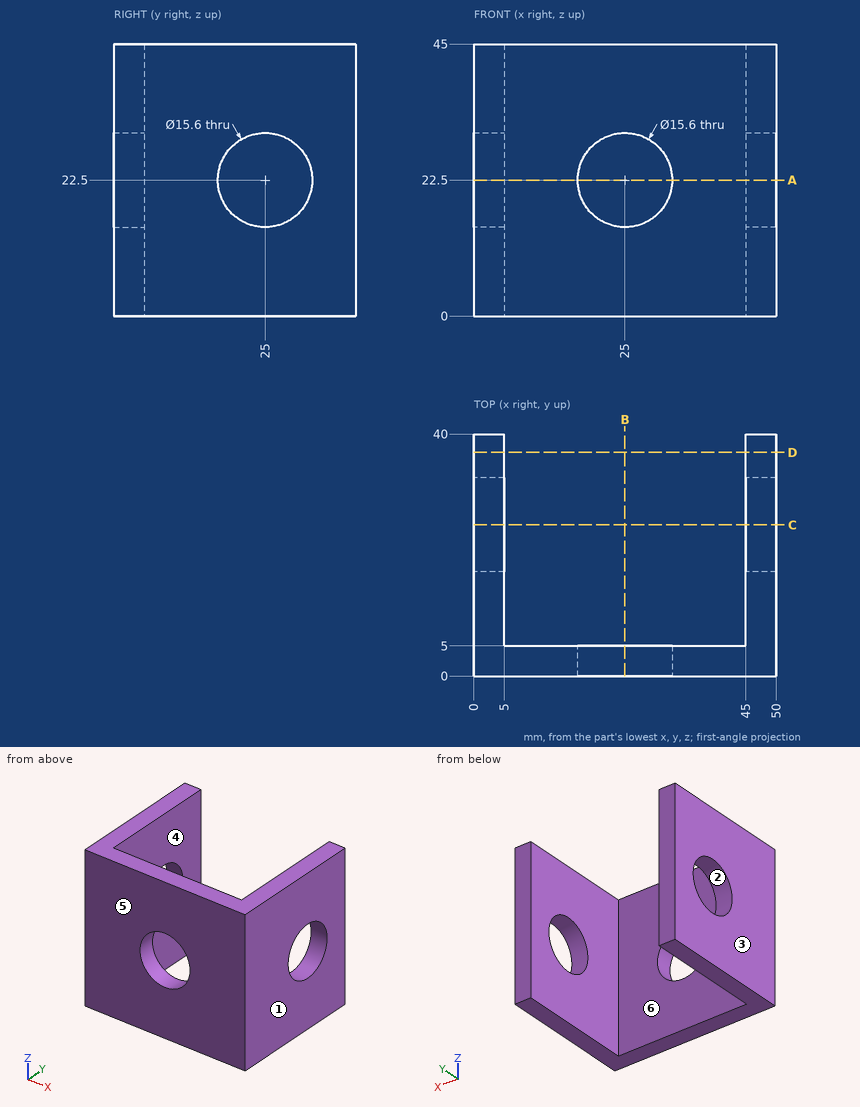
Design review of the part shown in the three views and the two pictorial views. Dimensions are in mm from the part's minimum x, y and z. A direction names the side the tool comes from. Round coordinates to 2 decimals unless told otherwise and drop trailing zeros. Write each loop counter-clockwise with the first axis right and the second up, starting at its lowest first coordinate (ties: lowest second). Pieces come first, ordered by that corner, then holes. Notation, with made-up numbers: M 64.25,-18 L 78.25,-18 A28 cw 78.25,8 Z; hole C -5.75,16.5 d10. An arc over 180 degrees is marked long. One line per item, written item: value. Start each with the question number.
1. Draft analysis for pull direction X (two halves, no side actions). For the marked faces 1, 2, 3 and 4, state which applies: pulls with the +X half, pulls with the -X half, needs draft (parallel to the pull), parting line crosses it, or undercut.
2. Take a section at D-D on y = 37. State the section outline as (x, z) points, then the cut area to 3 significant figures.
3. Take a section at C-C on y = 25. State the section outline as (x, z) points.
4. Take a section at B-B on x = 25. State the section outline as (y, z) points, then the cut area to 3 significant figures.
5. To check wall thickness, follow probe 1 along X at (y, z) = (21, 2); probe 2 along X at (y, z) = (1.8, 22.5); probe 3 along Z at (x, y) = (25, 1.4). State the ranges of each line that lie inside material, in increasing order. Write a range as from..to.
6. Take a section at A-A on z = 22.5. State the section outline as (x, y) points.
7. For the marked faces 5 and 6, list the 3-axis set-ups (+Z, -Z, +X, -X, +Y, -Y) from which the entire face can be reached by the end or side of a thin tool; tool diameter is ignored.
Computed:
1. face 1: pulls with the +X half
1. face 2: needs draft
1. face 3: pulls with the -X half
1. face 4: undercut
2. outline: M 0,0 L 5,0 L 5,45 L 0,45 Z; M 45,0 L 50,0 L 50,45 L 45,45 Z
2. area: 450 mm²
3. outline: M 0,0 L 5,0 L 5,14.7 L 0,14.7 Z; M 0,30.3 L 5,30.3 L 5,45 L 0,45 Z; M 45,0 L 50,0 L 50,14.7 L 45,14.7 Z; M 45,30.3 L 50,30.3 L 50,45 L 45,45 Z
4. outline: M 0,0 L 5,0 L 5,14.7 L 0,14.7 Z; M 0,30.3 L 5,30.3 L 5,45 L 0,45 Z
4. area: 147 mm²
5. probe 1: x = 0..5, 45..50
5. probe 2: x = 0..17.2, 32.8..50
5. probe 3: z = 0..14.7, 30.3..45
6. outline: M 0,0 L 17.2,0 L 17.2,5 L 5,5 L 5,17.2 L 0,17.2 Z; M 0,32.8 L 5,32.8 L 5,40 L 0,40 Z; M 32.8,0 L 50,0 L 50,17.2 L 45,17.2 L 45,5 L 32.8,5 Z; M 45,32.8 L 50,32.8 L 50,40 L 45,40 Z
7. face 5: +Z, -Z, +X, -X, -Y
7. face 6: +Z, -Z, +Y
